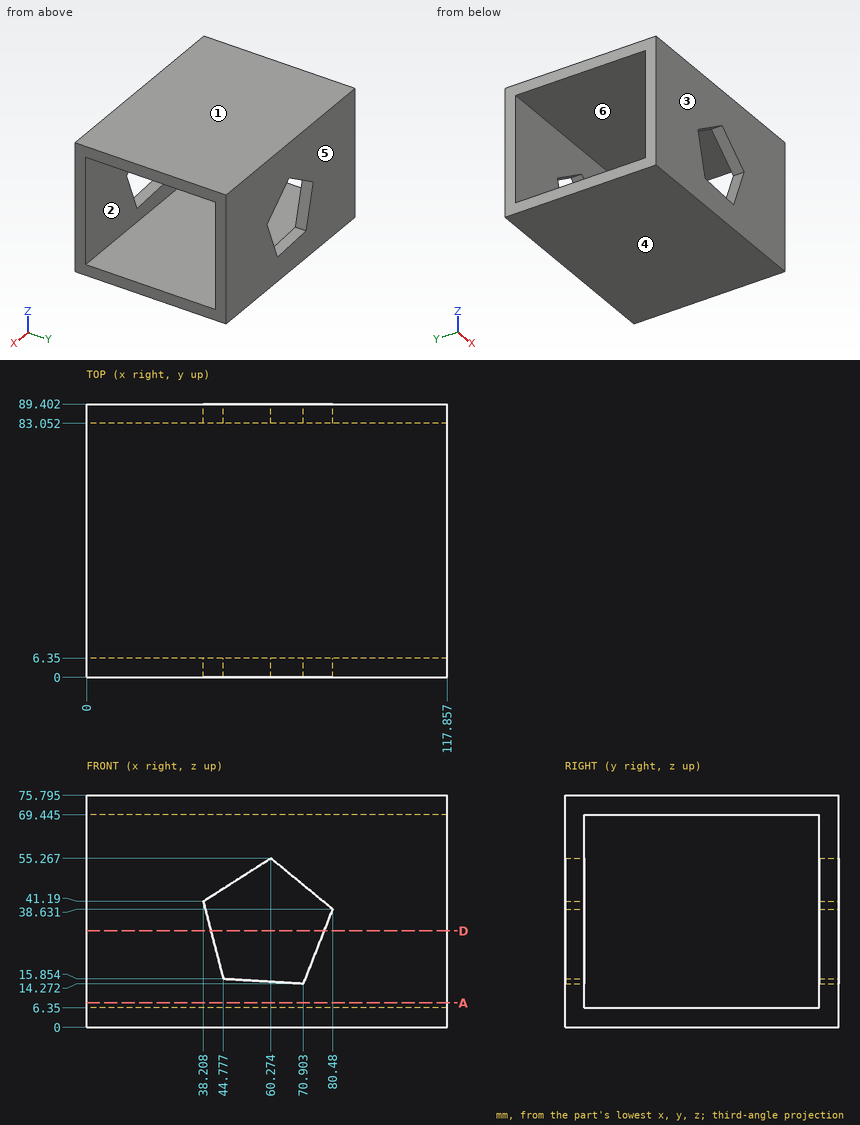
Input: dimensioned drawing with shaded views. Units: mm. Origin: part minimum x, y, z. A direction names the side the tool comes from. Round coordinates to 2 decimals unless told otherwise and drop trailing zeros. Loops run counter-clockwise (first coordinate to the right, second up) from the corner with the lowest first, then second, coordinate; pieces in that order, holes last. Notation, with made-up numbers: (74.25, 88.5) -> (127.25, 88.5) arc R15 ccw to (127.25, 116.5) -> close; hole circle Ø9 at (3.25, -7). An arc over 180 degrees is marked (long way). Use one line per item in the form item = value. Start each with the question number.
1) Line query: L1, parallel to Y at x = 18.5, z = 25.5. Output: solid intervals per line, ascending.
2) First-contact query: P1, Ø2, axis at y = 26, z = 8, coming from the -X side. Flat tip, straight axial feed; report the tip coordinate or a pass-through.
3) Draft query along Z for the marked faces 1, 2, 3 and 4. Return one class per face: released by +Z, released by -Z, zero draft, split by the parting line, or undercut.
4) Access query for the marked faces 5 and 6. Directions: +Z, -Z, +X, -X, +Y, -Y. A direction counts if a zero-diameter tool reaches every point of the face in a straight line with its end or side. Return the directions, or none.
5) Section D-D on z = 31.5. Output: boundary loops of the cut face in (x, y).
6) Section A-A on z = 8. Output: boundary loops of the cut face in (x, y).
Response:
q1.L1 = 0 to 6.35, 83.05 to 89.4
q2.P1 = through
q3.face_1 = released by +Z
q3.face_2 = undercut
q3.face_3 = zero draft
q3.face_4 = released by -Z
q4.face_5 = +Z, -Z, +X, -X, +Y
q4.face_6 = +X, -X
q5.outline = (0, 0) -> (40.72, 0) -> (40.72, 6.35) -> (0, 6.35) -> close; (0, 83.05) -> (40.72, 83.05) -> (40.72, 89.4) -> (0, 89.4) -> close; (77.68, 0) -> (117.86, 0) -> (117.86, 6.35) -> (77.68, 6.35) -> close; (77.68, 83.05) -> (117.86, 83.05) -> (117.86, 89.4) -> (77.68, 89.4) -> close
q6.outline = (0, 0) -> (117.86, 0) -> (117.86, 6.35) -> (0, 6.35) -> close; (0, 83.05) -> (117.86, 83.05) -> (117.86, 89.4) -> (0, 89.4) -> close
